CAD build for the part. Positions are in the model's coordinates, mm. A direction names the side the tool comes from. Give positions to 0.01 mm unless a question says otherwise; leave off trailing zeros. Loops run counter-clockwise (first coordinate to the right, second up) from the corner with the lowest first, then second, coordinate; pieces in that order, holes last.
```python
from build123d import *

# Parameters (mm, degrees)
SKETCH1_R           = 5.5
SKETCH1_R_2         = 2.75
BOSS_EXTRUDE1_DEPTH = 16
BOSS_EXTRUDE2_START = 1.5
SKETCH2_R           = 5.5
SKETCH2_R_2         = 1
BOSS_EXTRUDE2_DEPTH = 1.5
SKETCH3_R           = 5.5
SKETCH3_R_2         = 4.65
BOSS_EXTRUDE3_DEPTH = 50
CHAMFER1_SIZE       = 2
FILLET1_R           = 1


with BuildPart() as part:
    # Sketch1 → Boss-Extrude1 (new body)
    with BuildSketch(Plane(origin=(0, 0, 0), x_dir=(1, 0, 0), z_dir=(0, 1, 0))):
        with Locations(Location((0, 0, 0), (0, 0, 270))):
            Circle(SKETCH1_R)
        with Locations(Location((0, 0, 0), (0, 0, 270))):
            Circle(SKETCH1_R_2, mode=Mode.SUBTRACT)
    extrude(amount=BOSS_EXTRUDE1_DEPTH)

    # Sketch2 → Boss-Extrude2 (add)
    with BuildSketch(Plane.XZ.offset(BOSS_EXTRUDE2_START)):
        with Locations(Location((0, 0, 0), (0, 0, 270))):
            Circle(SKETCH2_R)
        with Locations(Location((0, 0, 0), (0, 0, 270))):
            Circle(SKETCH2_R_2, mode=Mode.SUBTRACT)
    extrude(amount=-BOSS_EXTRUDE2_DEPTH)

    # Sketch3 → Boss-Extrude3 (add)
    with BuildSketch(Plane(origin=(0, 16, 0), x_dir=(1, 0, 0), z_dir=(0, 1, 0))):
        with Locations(Location((0, 0, 0), (0, 0, 90))):
            Circle(SKETCH3_R)
        with Locations(Location((0, 0, 0), (0, 0, 270))):
            Circle(SKETCH3_R_2, mode=Mode.SUBTRACT)
    extrude(amount=BOSS_EXTRUDE3_DEPTH)

    # Chamfer1
    # the kernel refuses this chamfer: 2 mm, written as the material it adds along each edge
    with BuildSketch(Plane(origin=(0, 0, 0), x_dir=(0, 0, 1), z_dir=(-1, 0, 0))) as chamfer1_piece_1_section:
        Polygon((2.75 - CHAMFER1_SIZE, 0), (2.75, CHAMFER1_SIZE), (2.75, 0), align=None)
    chamfer1_piece_1 = revolve(axis=Axis((0, 0, 0), (0, 1, 0)), mode=Mode.PRIVATE)
    chamfer1_piece_1 = chamfer1_piece_1 - Plane(origin=(0, 1.131660662, 0), x_dir=(0, 0, -1), z_dir=(0, -1, 0)) * Cylinder(1, 11, mode=Mode.PRIVATE)
    add(chamfer1_piece_1)

    # Fillet1
    fillet1_edges = [part.edges().sort_by_distance(p)[0] for p in [
        (0, 16, -2.75),
    ]]
    fillet(fillet1_edges, radius=FILLET1_R)


solid = part.part
```
1. Probe line 1 along Z through (x, y) = (0, -0.9); line 2 along X through (y, z) = (9.75, 0); line 3 along X through (y, z) = (43, 0). List the from-to ranges inside material, lowest first.
Responses:
line 1: z = -5.5 to -1, 1 to 5.5
line 2: x = -5.5 to -2.75, 2.75 to 5.5
line 3: x = -5.5 to -4.65, 4.65 to 5.5
2. Saw through at D-D, the plane y = 7. List the corners of the cut face in (x, z).
Responses:
outline: circle Ø11 at (0, 0); hole circle Ø5.5 at (0, 0)
3. Drop flat-ended pins along their axis: pin 1 (2.5 mm diameter, centred on x = 0, z = 0, fed in from +Y); pin 2 (3 mm diameter, centred on x = 2, z = 0, fed in from +Y); pin 3 (1 mm diameter, centred on y = 14, z = 2.5, fed in from -X). Give the stop position or say it passes through.
Responses:
pin 1: stops at y = 0.5
pin 2: stops at y = 15.97
pin 3: stops at x = -5.12
4. Saw through at A-A, the plane x = 0. List the corners of the cut face in (y, z), and give its area (3 significant figures).
Responses:
outline: (-1.5, -5.5) - (66, -5.5) - (66, -4.65) - (16, -4.65) - (16, -3.75) arc R1 ccw to (15, -2.75) - (2, -2.75) - (0.25, -1) - (-1.5, -1) - close; (-1.5, 1) - (0.25, 1) - (2, 2.75) - (15, 2.75) arc R1 ccw to (16, 3.75) - (16, 4.65) - (66, 4.65) - (66, 5.5) - (-1.5, 5.5) - close
area: 190 mm2
5. Saw through at C-C, the plane y = 47. List the corners of the cut face in (x, z).
Responses:
outline: circle Ø11 at (0, 0); hole circle Ø9.3 at (0, 0)
6. Pull direction Z, two halves, no side cores. Call faces 1 (the face through (-1, 66, 5)), 2 (the face through (4, 16, 0)), 3 (the face through (-2.685, 8.409, -0.596)): released by +Z, released by -Z, zero draft, split by the parting line, or undercut.
Responses:
face 1: zero draft
face 2: undercut
face 3: undercut
7. Saw through at B-B, the plane z = 0. List the corners of the cut face in (x, y).
Responses:
outline: (-5.5, -1.5) - (-1, -1.5) - (-1, 0.25) - (-2.75, 2) - (-2.75, 15) arc R1 ccw to (-3.75, 16) - (-4.65, 16) - (-4.65, 66) - (-5.5, 66) - close; (1, -1.5) - (5.5, -1.5) - (5.5, 66) - (4.65, 66) - (4.65, 16) - (3.75, 16) arc R1 ccw to (2.75, 15) - (2.75, 2) - (1, 0.25) - close
8. Tool access for faces 4 (the face through (-1.15, -1.5, 0.08)), 5 (the face through (1.397, 40.65, 4.435)): list every direction of +Z, -Z, +X, -X, +Y, -Y with a clear straight run to the whole face (end or side of a thin tool).
Responses:
face 4: +Z, -Z, +X, -X, -Y
face 5: +Y
